Source: three-view drawing plus pictorial views. Frame: mm from the lowest corner of the part. A direction names the side the tool comes from. Coordinates: 2 decimals unless noted, no trailing zeros. Order: outer loops, then holes, each group sorted by start corner. A loop starts at its lowest first (then second) coordinate and runs counter-clockwise, first axis right, second up. Notation, with made-up numbers: (63, -25.75) -> (73, -25.75) arc R20 ccw to (73, 10.25) -> close; hole circle Ø10 at (-7, -21). An arc over 180 degrees is marked (long way). Use one line per item in the form item = value. Start each with the question number.
1) Section query B-B on z = 26.5. Output: boundary loops of the cut face in (x, y).
2) Section query A-A on x = 5.75. Output: boundary loops of the cut face in (y, z).
3) Section query C-C on x = 27.5. Output: boundary loops of the cut face in (y, z).
4) Section query D-D on z = 14.5. Output: boundary loops of the cut face in (x, y), then the cut area to 3 significant figures.
5) Pin query (flat end, axial travel): pin 1 (1 mm diameter, centred on x = 35, y = 6, fed in from +Z); pin 2 (5 mm diameter, centred on x = 60, z = 14, fed in from -Y); pin 3 (2.5 mm diameter, centred on x = 5.75, z = 3.5, fed in from +Y); pin 4 (4 mm diameter, centred on y = 3, z = 17.5, fed in from +X). Return the tip coordinate at first contact, or that it passes through.
6) Access query for the marked faces 1, 2 and 3. Directions: +Z, -Z, +X, -X, +Y, -Y. A direction counts if a zero-diameter tool reaches every point of the face in a straight line with its end or side. Return the directions, or none.
7) Ray query, line 1 along Z through (x, y) = (5.75, 8.65); line 2 along Z through (x, y) = (63.5, 8.75); line 3 along Y through (x, z) = (49, 3.75). Return the intervals inside material, ascending.
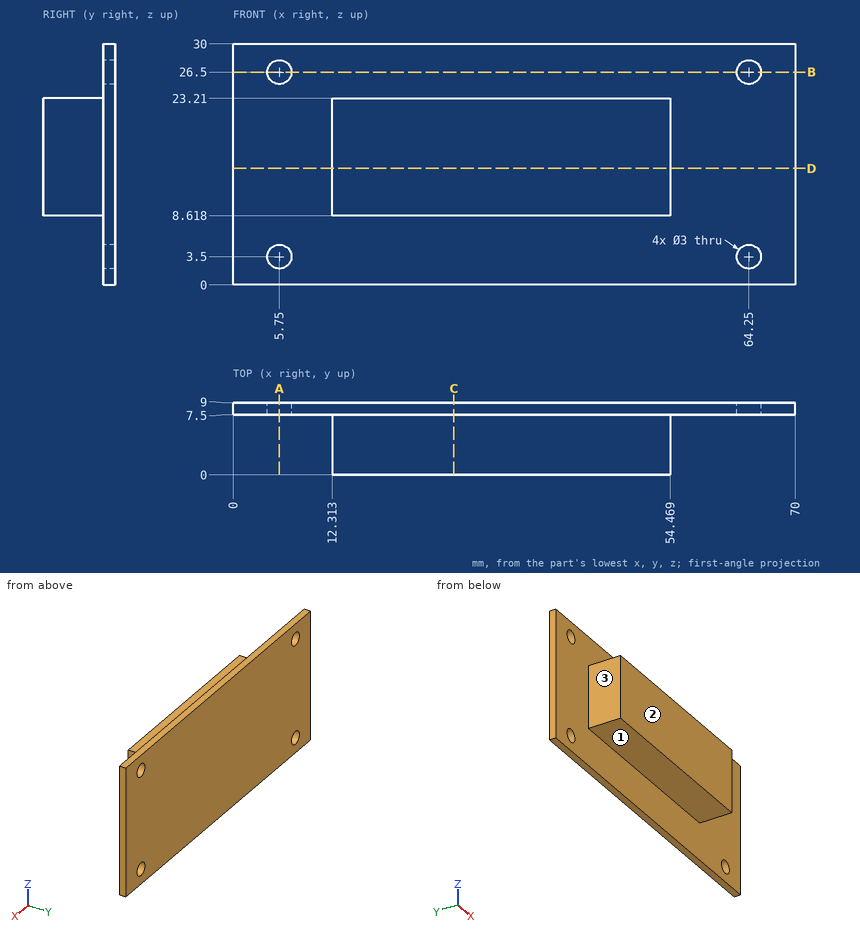
Answers below:
q1.outline = (0, 7.5) -> (4.25, 7.5) -> (4.25, 9) -> (0, 9) -> close; (7.25, 7.5) -> (62.75, 7.5) -> (62.75, 9) -> (7.25, 9) -> close; (65.75, 7.5) -> (70, 7.5) -> (70, 9) -> (65.75, 9) -> close
q2.outline = (7.5, 0) -> (9, 0) -> (9, 2) -> (7.5, 2) -> close; (7.5, 5) -> (9, 5) -> (9, 25) -> (7.5, 25) -> close; (7.5, 28) -> (9, 28) -> (9, 30) -> (7.5, 30) -> close
q3.outline = (0, 8.62) -> (7.5, 8.62) -> (7.5, 0) -> (9, 0) -> (9, 30) -> (7.5, 30) -> (7.5, 23.21) -> (0, 23.21) -> close
q4.outline = (0, 7.5) -> (12.31, 7.5) -> (12.31, 0) -> (54.47, 0) -> (54.47, 7.5) -> (70, 7.5) -> (70, 9) -> (0, 9) -> close
q4.area = 421 mm^2
q5.pin_1 = 23.21
q5.pin_2 = 7.5
q5.pin_3 = through
q5.pin_4 = 54.47
q6.face_1 = -Z, +X, -X, -Y
q6.face_2 = +Z, -Z, +X, -X, -Y
q6.face_3 = +Z, -Z, -X, -Y
q7.line_1 = 0 to 2, 5 to 25, 28 to 30
q7.line_2 = 0 to 2.2, 4.8 to 25.2, 27.8 to 30
q7.line_3 = 7.5 to 9
